```python
from build123d import *

# Parameters (mm, degrees)
SKETCH1_W           = 102
SKETCH1_H           = 132
BOSS_EXTRUDE2_DEPTH = 1
SKETCH2_W           = 3
SKETCH2_H           = 132
BOSS_EXTRUDE5_DEPTH = 3
SKETCH3_W           = 93
SKETCH3_H           = 126
BOSS_EXTRUDE6_DEPTH = 3
SKETCH4_R           = 7
CUT_EXTRUDE1_DEPTH  = 4


with BuildPart() as part:
    # Sketch1 → Boss-Extrude2 (new body)
    with BuildSketch(Plane(origin=(0, 0, 0), x_dir=(1, 0, 0), z_dir=(0, 1, 0))):
        Rectangle(SKETCH1_W, SKETCH1_H)
    extrude(amount=BOSS_EXTRUDE2_DEPTH)

    # Sketch2 → Boss-Extrude5 (add)
    with BuildSketch(Plane(origin=(0, 1, 0), x_dir=(1, 0, 0), z_dir=(0, 1, 0))):
        with Locations((-49.5, 0)):
            Rectangle(SKETCH2_W, SKETCH2_H)
    extrude(amount=BOSS_EXTRUDE5_DEPTH)

    # Sketch3 → Boss-Extrude6 (add)
    with BuildSketch(Plane(origin=(0, 1, 0), x_dir=(1, 0, 0), z_dir=(0, 1, 0))):
        with Locations((1.5, 0)):
            Rectangle(SKETCH3_W, SKETCH3_H)
    extrude(amount=BOSS_EXTRUDE6_DEPTH)

    # Sketch4 → Cut-Extrude1 (cut)
    with BuildSketch(Plane(origin=(0, 0, 0), x_dir=(1, 0, 0), z_dir=(0, 1, 0))):
        with Locations((24.75, 12.6)):
            Circle(SKETCH4_R)
        with Locations((24.75, -12.6)):
            Circle(SKETCH4_R)
        with Locations((24.75, 37.8)):
            Circle(SKETCH4_R)
        with Locations((24.75, -37.8)):
            Circle(SKETCH4_R)
    extrude(amount=CUT_EXTRUDE1_DEPTH, mode=Mode.SUBTRACT)


solid = part.part
```
Input: part model. Units: mm. Frame: model coordinates. A direction names the side the tool comes from. Coordinates: 2 decimals unless noted, no trailing zeros. Loops run counter-clockwise (first coordinate to the right, second up) from the corner with the lowest first, then second, coordinate; pieces in that order, holes last.
Q1. Contact query for flat-ended pins moving along their axis: pin 1 (22.5 mm diameter, centred on x = 24.75, z = 37.8, fed in from -Y); pin 2 (1.5 mm diameter, centred on y = 3, z = 7.5, fed in from +X); pin 3 (0.9 mm diameter, centred on x = -4.5, y = 2, fed in from +Z). Output: stop coordinate, or through.
Results are:
pin 1: stops at y = 0
pin 2: stops at x = 48
pin 3: stops at z = 63
Q2. Line query: line 1 along X through (y, z) = (1.3, 37.8); line 2 along Z through (x, y) = (24.75, 0.95); line 3 along Z through (x, y) = (24.75, 2.1). Output: solid intervals per line, ascending.
Results are:
line 1: x = -51 to -48, -45 to 17.75, 31.75 to 48
line 2: z = -66 to -44.8, -30.8 to -19.6, -5.6 to 5.6, 19.6 to 30.8, 44.8 to 66
line 3: z = -63 to -44.8, -30.8 to -19.6, -5.6 to 5.6, 19.6 to 30.8, 44.8 to 63
Q3. Section D-D, the plane z = -56. Return the cut outline in (x, y), and give its area (3 significant figures).
Results are:
outline: (-51, 0) - (51, 0) - (51, 1) - (48, 1) - (48, 4) - (-45, 4) - (-45, 1) - (-48, 1) - (-48, 4) - (-51, 4) - close
area: 390 mm2
Q4. Section C-C, the plane z = -12.6. Return the cut outline in (x, y).
Results are:
outline: (-51, 0) - (17.75, 0) - (17.75, 4) - (-45, 4) - (-45, 1) - (-48, 1) - (-48, 4) - (-51, 4) - close; (31.75, 0) - (51, 0) - (51, 1) - (48, 1) - (48, 4) - (31.75, 4) - close
Q5. Set-up query: faces 1 (the flat face through (1, 2, 63)), 2 (the flat face through (1, 2, -63)), 3 (the flat face through (-45, 2, 1)), 4 (the flat face through (48, 2, 1)). Return all of +Z, -Z, +X, -X, +Y, -Y with unobstructed straight access to the full face (end or side cutting, diameter ignored); none if empty.
Results are:
face 1: +Z, +X, +Y
face 2: -Z, +X, +Y
face 3: +Z, -Z, +Y
face 4: +Z, -Z, +X, +Y
Q6. Section B-B, the plane x = 24.75. Return the cut outline in (y, z).
Results are:
outline: (0, -66) - (1, -66) - (1, -63) - (4, -63) - (4, -44.8) - (0, -44.8) - close; (0, -30.8) - (4, -30.8) - (4, -19.6) - (0, -19.6) - close; (0, -5.6) - (4, -5.6) - (4, 5.6) - (0, 5.6) - close; (0, 19.6) - (4, 19.6) - (4, 30.8) - (0, 30.8) - close; (0, 44.8) - (4, 44.8) - (4, 63) - (1, 63) - (1, 66) - (0, 66) - close
Q7. Section A-A, the plane y = 1.65. Return the cut outline in (x, z).
Results are:
outline: (-51, -66) - (-48, -66) - (-48, 66) - (-51, 66) - close; (-45, -63) - (48, -63) - (48, 63) - (-45, 63) - close; hole circle Ø14 at (24.75, -37.8); hole circle Ø14 at (24.75, -12.6); hole circle Ø14 at (24.75, 12.6); hole circle Ø14 at (24.75, 37.8)
